Could you check a few things on this model? Use its own coordinates, in mm. Coordinates: 2 decimals unless noted, no trailing zeros. Order: outer loops, then holes, each group sorted by start corner. A loop starts at its lowest first (then second) coordinate and runs counter-clockwise, first axis right, second up. Notation, with made-up numbers: (-10, -0.5) -> (-1, -0.5) arc R17 ccw to (-1, 7.5) -> close; hole circle Ø5 at (86, 69). An arc over 180 degrees is marked (long way). Return JSON: item names as keys, results as strings. Group by question number.
from build123d import *

# Parameters (mm, degrees)
SKETCH1_R           = 120
BOSS_EXTRUDE1_DEPTH = 10
SKETCH2_R           = 10
BOSS_EXTRUDE2_DEPTH = 1500


with BuildPart() as part:
    # Sketch1 → Boss-Extrude1 (new body)
    with BuildSketch(Plane(origin=(0, 0, 0), x_dir=(1, 0, 0), z_dir=(0, 1, 0))):
        with Locations(Location((0, 0, 0), (0, 0, 270))):
            Circle(SKETCH1_R)
    extrude(amount=BOSS_EXTRUDE1_DEPTH)

    # Sketch2 → Boss-Extrude2 (add)
    with BuildSketch(Plane(origin=(0, 10, 0), x_dir=(1, 0, 0), z_dir=(0, 1, 0))):
        with Locations(Location((0, 100, 0), (0, 0, 270))):
            Circle(SKETCH2_R)
        with Locations(Location((-70, -75, 0), (0, 0, 270))):
            Circle(SKETCH2_R)
        with Locations(Location((70, -75, 0), (0, 0, 90))):
            Circle(SKETCH2_R)
    extrude(amount=BOSS_EXTRUDE2_DEPTH)


solid = part.part
Q1. I want a section at A-A on y = 1352. Please give me the cut outline in (x, z), and give its area (3 significant figures).
Q2. I want a section at C-C on x = 27.5. Please give me the cut outline in (y, z), and give its area (3 significant figures).
Q3. I want a section at B-B on z = -9. Please give me the cut outline in (x, y).
Q4. I need wall thicknesses on line 1 along Y through (x, z) = (52.5, 42.5); line 2 along Z through (x, y) = (70.5, 803); line 3 along Z through (x, y) = (72, 287). Which ranges of each line are inside material? Lowest first, please. Write a range as from..to.
Q5. I'm going to push flat-ended pins straight in: pin 1 Ø8 at (x, z) = (20.5, 6) entering from +Y; pin 2 Ø12 at (x, y) = (4.5, 344.5) entering from -Z; pin 3 Ø12 at (x, z) = (32.5, -94) entering from -Y; pin 4 Ø6 at (y, z) = (312.5, 73.5) entering from -X. Where does each tip first touch, or does it pass through?
Response values:
{
 "1": {"outline": "circle Ø20 at (-70, 75); circle Ø20 at (0, -100); circle Ø20 at (70, 75)", "area": "942 mm²"},
 "2": {"outline": "(0, -116.81) -> (10, -116.81) -> (10, 116.81) -> (0, 116.81) -> close", "area": "2,340 mm²"},
 "3": {"outline": "(-119.66, 0) -> (119.66, 0) -> (119.66, 10) -> (-119.66, 10) -> close"},
 "4": {"line 1": "y = 0..10", "line 2": "z = 65.01..84.99", "line 3": "z = 65.2..84.8"},
 "5": {"pin 1": "stops at y = 10", "pin 2": "stops at z = -110", "pin 3": "stops at y = 0", "pin 4": "stops at x = -80"}
}
